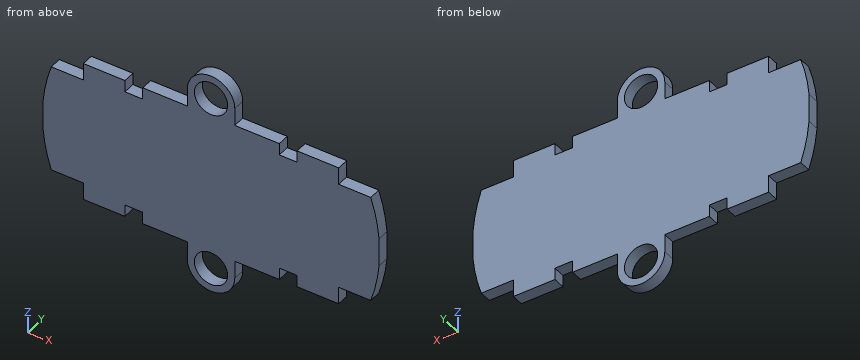
from build123d import *

# Parameters (mm, degrees)
SKETCH1_W               = 54.61
SKETCH1_H               = 23.114
SKETCH1_W_2             = 8.636
SKETCH1_H_2             = 3.683
BOSS_EXTRUDE1_DEPTH     = 2.54
CUT_EXTRUDE1_DEPTH      = 3.54
CUT_EXTRUDE1_DEPTH_BACK = 1
SKETCH3_R               = 3.556
BOSS_EXTRUDE2_DEPTH     = 2.54
SKETCH4_W               = 3.81
SKETCH4_H               = 2.54
CUT_EXTRUDE3_DEPTH      = 3.54


with BuildPart() as part:
    # Sketch1 → Boss-Extrude1 (new body)
    with BuildSketch(Plane(origin=(0, 0, 0), x_dir=(1, 0, 0), z_dir=(0, 1, 0))):
        Rectangle(SKETCH1_W, SKETCH1_H)
        with Locations((-31.623, 0)):
            Rectangle(SKETCH1_W_2, SKETCH1_H)
        with Locations((31.623, 0)):
            Rectangle(SKETCH1_W_2, SKETCH1_H)
        with Locations((0, -13.3985)):
            Rectangle(SKETCH1_W, SKETCH1_H_2)
        with Locations((0, 13.3985)):
            Rectangle(SKETCH1_W, SKETCH1_H_2)
    extrude(amount=BOSS_EXTRUDE1_DEPTH)

    # Sketch2 → Cut-Extrude1 (cut, two sides)
    with BuildSketch(Plane(origin=(0, 0, 0), x_dir=(1, 0, 0), z_dir=(0, 1, 0))) as cut_extrude1_sk:
        with BuildLine():
            Line((-36.068, 36.068), (-36.068, -3.1e-08))
            ThreePointArc((-36.068, -3.1e-08), (-25.503927395, 25.503927373), (0, 36.068))
            Line((0, 36.068), (-36.068, 36.068))
        make_face()
        with BuildLine():
            ThreePointArc((0, 36.068), (25.503927384, 25.503927384), (36.068, 0))
            Line((36.068, 0), (36.068, 36.068))
            Line((36.068, 36.068), (0, 36.068))
        make_face()
        with BuildLine():
            ThreePointArc((36.068, 0), (25.503927365, -25.503927403), (-5.3e-08, -36.068))
            Line((-5.3e-08, -36.068), (36.068, -36.068))
            Line((36.068, -36.068), (36.068, 0))
        make_face()
        with BuildLine():
            Line((-36.068, -3.1e-08), (-36.068, -36.068))
            Line((-36.068, -36.068), (-5.3e-08, -36.068))
            ThreePointArc((-5.3e-08, -36.068), (-25.503927391, -25.503927376), (-36.068, -3.1e-08))
        make_face()
    extrude(amount=CUT_EXTRUDE1_DEPTH, mode=Mode.SUBTRACT)
    extrude(cut_extrude1_sk.sketch, amount=-CUT_EXTRUDE1_DEPTH_BACK, mode=Mode.SUBTRACT)

    # Sketch3 → Boss-Extrude2 (add)
    with BuildSketch(Plane(origin=(0, 0, 0), x_dir=(1, 0, 0), z_dir=(0, 1, 0))):
        with BuildLine():
            Line((-5.08, 19.05), (-5.08, 15.24))
            Line((-5.08, 15.24), (5.08, 15.24))
            Line((5.08, 15.24), (5.08, 19.05))
            ThreePointArc((5.08, 19.05), (0, 24.13), (-5.08, 19.05))
        make_face()
        with Locations((0, 19.05)):
            Circle(SKETCH3_R, mode=Mode.SUBTRACT)
        with BuildLine():
            Line((-5.08, -19.05), (-5.08, -15.24))
            Line((-5.08, -15.24), (5.08, -15.24))
            Line((5.08, -15.24), (5.08, -19.05))
            ThreePointArc((5.08, -19.05), (0, -24.13), (-5.08, -19.05))
        make_face()
        with Locations((0, -19.05)):
            Circle(SKETCH3_R, mode=Mode.SUBTRACT)
    extrude(amount=BOSS_EXTRUDE2_DEPTH)

    # Sketch4 → Cut-Extrude3 (cut, through all)
    with BuildSketch(Plane(origin=(0, 0, 0), x_dir=(1, 0, 0), z_dir=(0, 1, 0))):
        with Locations((-16.51, 13.97)):
            Rectangle(SKETCH4_W, SKETCH4_H)
        with Locations((16.51, 13.97)):
            Rectangle(SKETCH4_W, SKETCH4_H)
        with Locations((-16.51, -13.97)):
            Rectangle(SKETCH4_W, SKETCH4_H)
        with Locations((16.51, -13.97)):
            Rectangle(SKETCH4_W, SKETCH4_H)
    extrude(amount=CUT_EXTRUDE3_DEPTH, mode=Mode.SUBTRACT)


solid = part.part
Work out the finished part from the listing and answer in its coordinate system (mm). Give positions to 0.01 mm unless a question says otherwise; leave off trailing zeros. Write each loop counter-clockwise with the first axis right and the second up, starting at its lowest first coordinate (ties: lowest second). Pieces come first, ordered by that corner, then holes.
Q1. Straight lines are drawn through the part: L1, parallel to Z at x = 0, y = 2.05; L2, parallel to X at y = 0.2, z = 13 (3 decimals); L3, parallel to Z at x = 2, y = 1.25. For each, find the intervals that lie inside material, in ascending order.
Answer:
L1: z = -24.13 to -22.61, -15.49 to 15.49, 22.61 to 24.13
L2: x = -27.305 to -18.415, -14.605 to 14.605, 18.415 to 27.305
L3: z = -23.72 to -21.99, -16.11 to 16.11, 21.99 to 23.72
Q2. The part is cut by section D-D on y = 1.9. State how many separate pieces and enclosed holes the cut face has, and give its area (3 significant figures).
Answer:
separate pieces: 1
enclosed holes: 2
area: 2,080 mm2
Q3. The part is cut by section A-A on x = 0. Give the vertices of the cut face in (y, z).
Answer:
outline: (0, -24.13) - (2.54, -24.13) - (2.54, -22.61) - (0, -22.61) - close; (0, -15.49) - (2.54, -15.49) - (2.54, 15.49) - (0, 15.49) - close; (0, 22.61) - (2.54, 22.61) - (2.54, 24.13) - (0, 24.13) - close
Q4. Given pin 1 (1.3 mm diameter, centred on y = 1.5, z = 14.5, fed in from -X) (3 decimals); pin 2 (1 mm diameter, centred on y = 1.5, z = -13.5, fed in from +X) (3 decimals); pin 3 (0.8 mm diameter, centred on y = 0.5, z = -16, fed in from +X), each flat-ended and moving along its own axis, determine where each tip first touches the part or whether it passes through.
Answer:
pin 1: stops at x = -27.305
pin 2: stops at x = 27.305
pin 3: stops at x = 5.08
Q5. The part is cut by section C-C on z = 21.5. Give the vertices of the cut face in (x, y), and give its area (3 significant figures).
Answer:
outline: (-4.45, 0) - (-2.58, 0) - (-2.58, 2.54) - (-4.45, 2.54) - close; (2.58, 0) - (4.45, 0) - (4.45, 2.54) - (2.58, 2.54) - close
area: 9.51 mm2
Q6. The part is cut by section B-B on z = 14. Give the vertices of the cut face in (x, y) (3 decimals).
Answer:
outline: (-27.305, 0) - (-18.415, 0) - (-18.415, 2.54) - (-27.305, 2.54) - close; (-14.605, 0) - (14.605, 0) - (14.605, 2.54) - (-14.605, 2.54) - close; (18.415, 0) - (27.305, 0) - (27.305, 2.54) - (18.415, 2.54) - close
